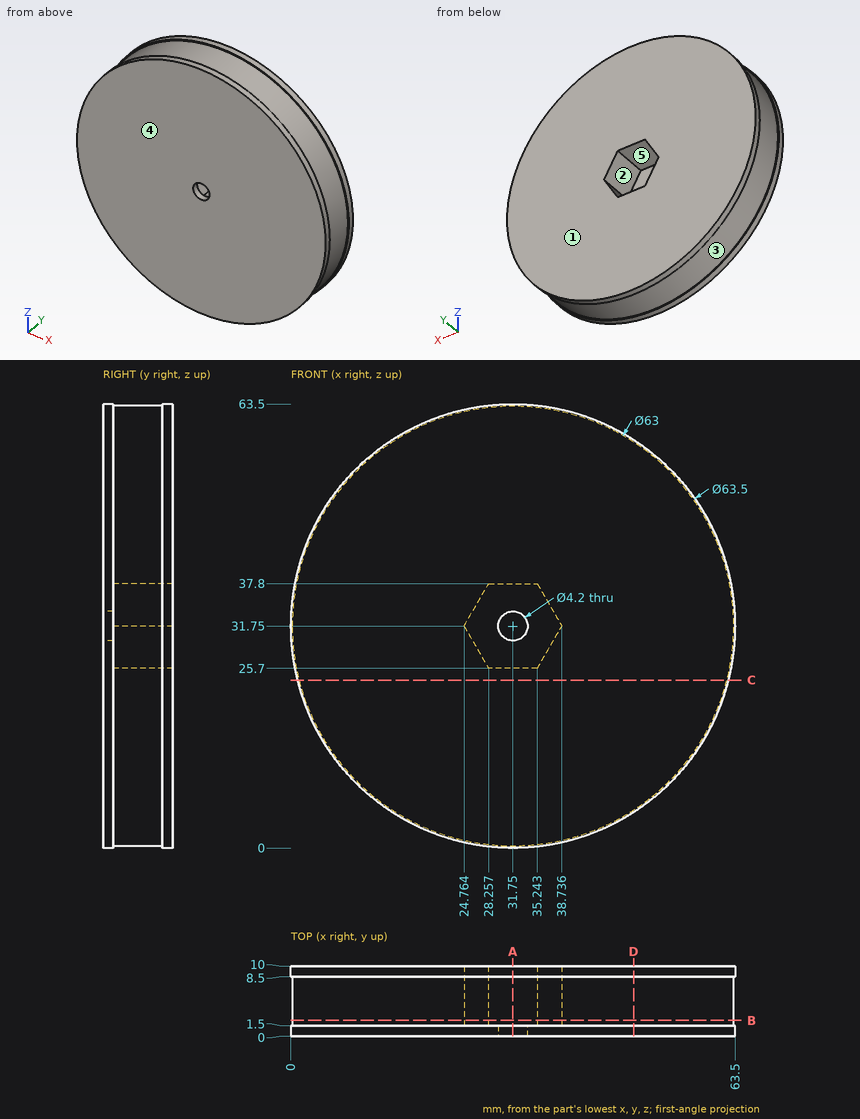
Verification items for this drawing (mm, ordinates from the low corner). A direction names the side the tool comes from. Coordinates: 2 decimals unless noted, no trailing zeros. Write each loop counter-clockwise with the first axis right and the second up, starting at its lowest first coordinate (ties: lowest second). Pieces come first, ordered by that corner, then holes. Notation, with made-up numbers: M 30,71.5 L 58,71.5 A26 ccw 58,105.5 Z; hole C 13.5,33.25 d2. An arc over 180 degrees is marked long. Use one line per item in the form item = value. Start each with the question number.
1) Section check D-D on x = 49. Enter the section's corners in (y, z) (3 decimals).
2) Section check B-B on y = 2.25. Enter the section's corners in (x, z), and give its area (3 significant figures).
3) Section check C-C on z = 24. Enter the section's corners in (x, y).
4) Release check for a two-part mould opening along Y. For the marked faces 3, 4 and 5 record: pulls with the +Y half, pulls with the -Y half, needs draft (parallel to the pull), parting line crosses it, or undercut.
5) Thickness scan on probe 1 along X at (y, z) = (1, 31.75); probe 2 along Z at (x, y) = (34, 9.25). Record the ranges inside material, lowest first. Write a range as from..to.
6) Set-up check for the marked faces 1 and 2: record each of +Z, -Z, +X, -X, +Y, -Y from which the full face is reachable in a straight line by a thin tool's end or side.
7) Section check A-A on x = 31.75. Enter the section's corners in (y, z).
8) Go/stop test with flat-tipped pins: pin 1 Ø3.5 at (x, z) = (34.5, 32.5) entering from +Y; pin 2 Ø1 at (y, z) = (2.5, 47) entering from +X; pin 3 Ø3.5 at (x, y) = (32.5, 7.5) entering from +Z; pin 4 Ø4 at (x, z) = (31.75, 31.75) entering from -Y. Record where each tip stops, or that it passes through.
Responses:
q1.outline = M 0,5.095 L 1.5,5.095 L 1.5,5.393 L 8.5,5.393 L 8.5,5.095 L 10,5.095 L 10,58.405 L 8.5,58.405 L 8.5,58.107 L 1.5,58.107 L 1.5,58.405 L 0,58.405 Z
q2.outline = C 31.75,31.75 d63; hole M 24.76,31.75 L 28.26,25.7 L 35.24,25.7 L 38.74,31.75 L 35.24,37.8 L 28.26,37.8 Z
q2.area = 2,990 mm2
q3.outline = M 0.96,0 L 62.54,0 L 62.54,1.5 L 62.28,1.5 L 62.28,8.5 L 62.54,8.5 L 62.54,10 L 0.96,10 L 0.96,8.5 L 1.22,8.5 L 1.22,1.5 L 0.96,1.5 Z
q4.face_3 = undercut
q4.face_4 = pulls with the -Y half
q4.face_5 = needs draft
q5.probe_1 = 0..29.65, 33.85..63.5
q5.probe_2 = 0.08..25.7, 37.8..63.42
q6.face_1 = +Z, -Z, +X, -X, +Y
q6.face_2 = +Y
q7.outline = M 0,0 L 1.5,0 L 1.5,0.25 L 8.5,0.25 L 8.5,0 L 10,0 L 10,25.7 L 1.5,25.7 L 1.5,29.65 L 0,29.65 Z; M 0,33.85 L 1.5,33.85 L 1.5,37.8 L 10,37.8 L 10,63.5 L 8.5,63.5 L 8.5,63.25 L 1.5,63.25 L 1.5,63.5 L 0,63.5 Z
q8.pin_1 = 1.5
q8.pin_2 = 59.58
q8.pin_3 = 63.5
q8.pin_4 = through
